Design review of the part built by this model. Coordinates are the model's own, in mm. A direction names the side the tool comes from. Give positions to 0.01 mm unless a question says otherwise; leave off trailing zeros. Order: outer loops, then holes, each group sorted by start corner. A loop starts at its lowest first (then second) coordinate and runs counter-clockwise, first axis right, second up. Notation, with made-up numbers: M 82,72.5 L 132,72.5 A35 ccw 132,109.5 Z; hole C -16.5,-31.75 d10. An arc over 180 degrees is marked long. Answer as a JSON object with one key per item and string values.
from build123d import *

# Parameters (mm, degrees)
F0_R          = 27.233083
F1_DEPTH      = 101.6
F1_DEPTH_BACK = 101.6
F2_W          = 63.5
F2_H          = 63.5
F2_R          = 27.233083
F3_DEPTH      = 25.4
F5_W          = 63.5
F5_H          = 63.5
F6_DEPTH      = 25.4
F4_R          = 22.225
F7_DEPTH      = 203.2


with BuildPart() as f1:
    # F0 (on Front) → F1 (new body, two sides)
    with BuildSketch(Plane.XZ) as f1_sk:
        Circle(F0_R)
    extrude(amount=F1_DEPTH)
    extrude(f1_sk.sketch, amount=-F1_DEPTH_BACK)

    # F2 (on face) → F3 (join)
    with BuildSketch(Plane.XZ.offset(101.6)):
        with Locations((0.706917, 0.563083)):
            Rectangle(F2_W, F2_H)
        Circle(F2_R, mode=Mode.SUBTRACT)
    extrude(amount=-F3_DEPTH)

    # F5 (on face) → F6 (join)
    with BuildSketch(Plane(origin=(0, 101.6, 0), x_dir=(-1, 0, 0), z_dir=(0, 1, 0))):
        with Locations((-0.664903, 0.443074)):
            Rectangle(F5_W, F5_H)
    extrude(amount=-F6_DEPTH)

    # F4 (on face) → F7 (cut)
    with BuildSketch(Plane.XZ.offset(101.6)):
        Circle(F4_R)
    extrude(amount=-F7_DEPTH, mode=Mode.SUBTRACT)


solid = f1.part
(1) We need section D-D (z = -25). Write out the cut boundary in (x, y), plus the area to 3 significant figures.
Checked values:
{"outline": "M -31.09,76.2 L -10.8,76.2 L -10.8,-76.2 L -31.04,-76.2 L -31.04,-101.6 L 32.46,-101.6 L 32.46,-76.2 L 10.8,-76.2 L 10.8,76.2 L 32.41,76.2 L 32.41,101.6 L -31.09,101.6 Z", "area": "6,520 mm^2"}
(2) Draft analysis for pull direction Y (two halves, no side actions). For faces 1 (the flat face through (29, 76.2, 1)), 2 (the flat face through (1, 89, 32.193)), 3 (the flat face through (22, 101.6, 8)), state which applies: +Y half, -Y half, draft (parallel to the pull), parting line (faces both ways), or undercut.
Checked values:
{"face 1": "undercut", "face 2": "draft", "face 3": "+Y half"}
(3) We need section A-A (x = 0). Write out the cut boundary in (y, z) (3 decimals), plus the area to 3 significant figures.
Checked values:
{"outline": "M -101.6,-31.187 L -76.2,-31.187 L -76.2,-27.233 L 76.2,-27.233 L 76.2,-31.307 L 101.6,-31.307 L 101.6,-22.225 L -101.6,-22.225 Z; M -101.6,22.225 L 101.6,22.225 L 101.6,32.193 L 76.2,32.193 L 76.2,27.233 L -76.2,27.233 L -76.2,32.313 L -101.6,32.313 Z", "area": "2,490 mm^2"}
(4) We need section B-B (z = 0). Write out the cut boundary in (x, y) (3 decimals), plus the area to 3 significant figures.
Checked values:
{"outline": "M -31.085,76.2 L -27.233,76.2 L -27.233,-76.2 L -31.043,-76.2 L -31.043,-101.6 L -22.225,-101.6 L -22.225,101.6 L -31.085,101.6 Z; M 22.225,-101.6 L 32.457,-101.6 L 32.457,-76.2 L 27.233,-76.2 L 27.233,76.2 L 32.415,76.2 L 32.415,101.6 L 22.225,101.6 Z", "area": "2,490 mm^2"}
(5) We need section C-C (y = -57). Write out the cut boundary in (x, z) (3 decimals), plus the area to 3 significant figures.
Checked values:
{"outline": "C 0,0 d54.466; hole C 0,0 d44.45", "area": "778 mm^2"}
(6) Tool access review of faces 4 (the flat face through (0, -76.2, 29)), 5 (the flat face through (32.457, -89, 0)): name each direction out of +Z, -Z, +X, -X, +Y, -Y from which nothing blocks a thin tool from reaching the whole face with its end or side.
Checked values:
{"face 4": "none", "face 5": "+Z, -Z, +X, +Y, -Y"}
(7) To check wall thickness, follow L1, parallel to Y at x = 28.5, z = -29; L2, parallel to Z at x = 0, y = -43.5 (3 decimals); L3, parallel to Z at x = 23, y = 83.5. State the ranges of each line that lie inside material, in increasing order. Write a range as from..to.
Checked values:
{"L1": "y = -101.6..-76.2, 76.2..101.6", "L2": "z = -27.233..-22.225, 22.225..27.233", "L3": "z = -31.31..32.19"}
(8) Insertion check: pin 1 (7.5 mm diameter, centred on x = -4, y = 93, fed in from +Z); pin 2 (12 mm diameter, centred on y = -75, z = -17, fed in from -X); pin 3 (1 mm diameter, centred on x = -11, y = 8.5, fed in from +Z). Each pin has a flat end and moves straight along its axis. Give the tip position at first contact, or say it passes through.
Checked values:
{"pin 1": "stops at z = 32.19", "pin 2": "stops at x = -31.04", "pin 3": "stops at z = 25.13"}
